The model under review builds one solid part; all positions refer to its coordinate system, in mm. Round coordinates to 2 decimals unless told otherwise and drop trailing zeros. Write each loop counter-clockwise with the first axis right and the second up, starting at its lowest first coordinate (ties: lowest second). Pieces come first, ordered by that corner, then holes. Notation, with made-up numbers: (54, 89.5) -> (63, 89.5) arc R18 ccw to (63, 100.5) -> close; hole circle Ø1 at (-13.5, 7.25). An arc over 180 degrees is marked (long way). Answer as a JSON object with one key per item and string values. Group by question number.
1) We need section C-C, the plane z = 2.1. Write out the cut boundary in (x, y).
2) To check wall thickness, follow probe 1 along X at (y, z) = (-18, 2.3); probe 2 along Y at (x, z) = (-51.5, 0.6); probe 3 along Y at (x, z) = (37.5, 0.2). State the ranges of each line that lie inside material, in increasing order. Write a range as [from, to].
3) We need section B-B, the plane y = 17. Write out the cut boundary in (x, z), then the cut area to 3 significant figures.
4) Mouldability with a two-part tool opening along X and no side actions: class faces 1 (the flat face through (1, -3, 2.5)), 2 (the flat face through (-92.07, -8.54, 1.23)), 3 (the cylindrical face through (1.919, 22.356, 1.232)), 4 (the cylindrical face through (73.98, -24.236, 1.232)) as pulls with the +X half, pulls with the -X half, needs draft (parallel to the pull), parting line crosses it, or undercut.
5) We need section A-A, the plane x = 33. Write out the cut boundary in (y, z).
6) Insertion check: pin 1 Ø0.8 at (x, z) = (18.5, 1.5) entering from +Y; pin 2 Ø1.5 at (x, y) = (29, 32) entering from -Z. Each pin has a flat end and moves straight along its axis. Give the tip position at first contact, or say it passes through.
7) We need section D-D, the plane y = -10. Write out the cut boundary in (x, z).
from build123d import *

# Parameters (mm, degrees)
F0_R     = 5
F1_DEPTH = 2.5


with BuildPart() as f1:
    # F0 (on Top) → F1 (new body)
    with BuildSketch(Plane.XY):
        with BuildLine():
            Line((-97.139122, -17.320508), (-97.139122, -33.320508))
            Line((-97.139122, -33.320508), (-63.639122, -33.320508))
            Line((-63.639122, -33.320508), (69.360878, -33.320508))
            Line((69.360878, -33.320508), (102.860878, -33.320508))
            Line((102.860878, -33.320508), (102.860878, -17.320508))
            Line((102.860878, -17.320508), (92.860878, 0))
            ThreePointArc((92.860878, 0), (2.860878, 42.320195), (-87.139122, 0))
            Line((-87.139122, 0), (-97.139122, -17.320508))
        make_face()
        with Locations((-63.639122, -22.320508)):
            Circle(F0_R, mode=Mode.SUBTRACT)
        with Locations((69.360878, -22.320508)):
            Circle(F0_R, mode=Mode.SUBTRACT)
        with BuildLine():
            ThreePointArc((-59.139122, 0), (2.860878, 22.360343), (64.860878, 0))
            Line((64.860878, 0), (-59.139122, 0))
        make_face(mode=Mode.SUBTRACT)
    extrude(amount=F1_DEPTH)


solid = f1.part
Here are the results:
{
 "1": {"outline": "(-97.14, -33.32) -> (102.86, -33.32) -> (102.86, -17.32) -> (92.86, 0) arc R116.86 ccw to (-87.14, 0) -> (-97.14, -17.32) -> close; hole circle Ø10 at (-63.64, -22.32); hole (-59.14, 0) -> (64.86, 0) arc R97.14 ccw to start; hole circle Ø10 at (69.36, -22.32)"},
 "2": {"probe 1": "x = [-97.14, -66.16], [-61.12, 66.84], [71.88, 102.86]", "probe 2": "y = [-33.32, 0], [5.72, 28.91]", "probe 3": "y = [-33.32, 0], [15.97, 37.07]"},
 "3": {"outline": "(-69.78, 0) -> (-28.96, 0) -> (-28.96, 2.5) -> (-69.78, 2.5) -> close; (34.68, 0) -> (75.5, 0) -> (75.5, 2.5) -> (34.68, 2.5) -> close", "area": "204 mm^2"},
 "4": {"face 1": "needs draft", "face 2": "pulls with the -X half", "face 3": "undercut", "face 4": "undercut"},
 "5": {"outline": "(-33.32, 0) -> (0, 0) -> (0, 2.5) -> (-33.32, 2.5) -> close; (17.57, 0) -> (38.37, 0) -> (38.37, 2.5) -> (17.57, 2.5) -> close"},
 "6": {"pin 1": "stops at y = 41.32", "pin 2": "stops at z = 0"},
 "7": {"outline": "(-92.91, 0) -> (98.63, 0) -> (98.63, 2.5) -> (-92.91, 2.5) -> close"}
}
